Input: part model. Units: mm. Frame: model coordinates. Face numbers are marked on the shaded views. A direction names the side the tool comes from. Coordinates: 2 decimals unless noted, no trailing zeros. Order: outer loops, then holes, each group sorted by start corner. A loop starts at its lowest first (then second) coordinate and runs counter-clockwise, first axis right, second up.
from build123d import *

# Parameters (mm, degrees)
BASE_FLANGE1_DEPTH           = 3.175
EDGE_FLANGE1_DEPTH           = 16.378
EDGE_FLANGE2_STRIP_W         = 14.1732
EDGE_FLANGE2_STRIP_H         = 3.175
EDGE_FLANGE2_STRIP_CUT_DEPTH = 16.378
EDGE_FLANGE2_DEPTH           = 16.378
M5_CLEARANCE_HOLE1_D         = 5.5
M6_CLEARANCE_HOLE1_D         = 6.6
FILLET1_R                    = 2.54
M3_CLEARANCE_HOLE1_D         = 3.4


# Sheet-metal steps are written as plain solids
with BuildPart() as part:
    # Sketch1 → Base-Flange1 (new body)
    with BuildSketch(Plane.XY):
        Polygon((-22.215900005, -29.184600001), (-22.215900005, -69.692600001), (-5.837899995, -69.692600001), (-5.837899995, -45.562600001), (61.9125, -45.562600001), (61.9125, -29.184600001), align=None)
    extrude(amount=-BASE_FLANGE1_DEPTH)

    # Edge-Flange1 section (across the edge) → Edge-Flange1 (add)
    with BuildSketch(Plane(origin=(62.6491, -45.562600001, 0), x_dir=(-1, 0, 0), z_dir=(0, 1, 0))):
        with BuildLine():
            Line((-3.175, 0.7366), (-3.175, 32.0779))
            Line((-3.175, 32.0779), (0, 32.0779))
            Line((0, 32.0779), (0, 0.7366))
            ThreePointArc((0, 0.7366), (0.215745145, 0.215745145), (0.7366, 0))
            Line((0.7366, 0), (0.7366, -3.175))
            ThreePointArc((0.7366, -3.175), (-2.029318885, -2.029318885), (-3.175, 0.7366))
        make_face()
    extrude(amount=EDGE_FLANGE1_DEPTH)

    # Edge-Flange2 strip (across the edge) → Edge-Flange2 strip cut (cut)
    with BuildSketch(Plane(origin=(65.8241, -29.184600001, 32.0779), x_dir=(0, 0, -1), z_dir=(0, -1, 0))):
        with Locations((-6.35, -1.5875)):
            Rectangle(EDGE_FLANGE2_STRIP_W, EDGE_FLANGE2_STRIP_H)
    extrude(amount=EDGE_FLANGE2_STRIP_CUT_DEPTH, mode=Mode.SUBTRACT)

    # Edge-Flange2 section (across the edge) → Edge-Flange2 (add)
    with BuildSketch(Plane(origin=(65.8241, -29.184600001, 32.0779), x_dir=(0, 0, -1), z_dir=(0, -1, 0))):
        with BuildLine():
            Line((-3.175, 0.7366), (-3.175, 60.325))
            Line((-3.175, 60.325), (0, 60.325))
            Line((0, 60.325), (0, 0.7366))
            ThreePointArc((0, 0.7366), (0.215745145, 0.215745145), (0.7366, 0))
            Line((0.7366, 0), (0.7366, -3.175))
            ThreePointArc((0.7366, -3.175), (-2.029318885, -2.029318885), (-3.175, 0.7366))
        make_face()
    extrude(amount=EDGE_FLANGE2_DEPTH)

    # M5 Clearance Hole1 (through all)
    with Locations(Plane.XY.offset(35.2529)):
        with Locations((119.7991, -37.373600001)):
            Hole(M5_CLEARANCE_HOLE1_D / 2)

    # M6 Clearance Hole1 (through all)
    with Locations(Plane.XY):
        with Locations((-14.0269, -61.865600001)):
            Hole(M6_CLEARANCE_HOLE1_D / 2)

    # Fillet1
    fillet1_edges = [part.edges().sort_by_distance(p)[0] for p in [
        (-22.215900005, -69.692600001, -1.5875),
        (-22.215900005, -29.184600001, -1.5875),
        (-5.837899995, -45.562600001, -1.5875),
        (-5.837899995, -69.692600001, -1.5875),
        (126.1491, -29.184600001, 33.6654),
        (126.1491, -45.562600001, 33.6654),
    ]]
    fillet(fillet1_edges, radius=FILLET1_R)

    # M3 Clearance Hole1 (through all)
    with Locations(Plane.XY.offset(35.2529)):
        with Locations((96.0232, -37.423600001)):
            Hole(M3_CLEARANCE_HOLE1_D / 2)


solid = part.part
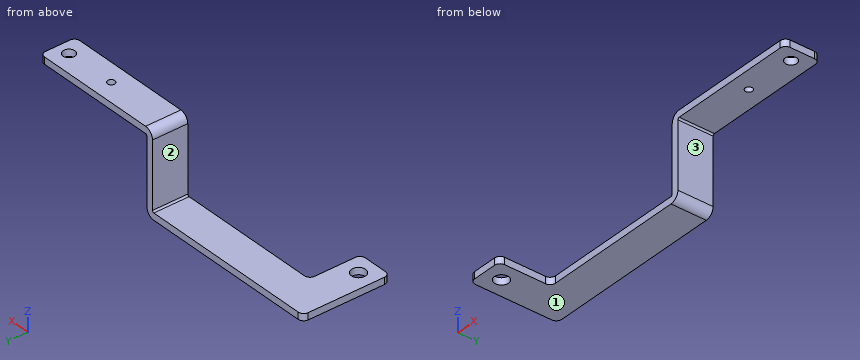
Item 1: Cut plane B-B on z = 25. Return loops of the section in (x, y).
Response values:
outline: (62.65, -45.56) - (65.82, -45.56) - (65.82, -29.18) - (62.65, -29.18) - close
Item 2: Pin query (flat end, axial travel): pin 1 Ø1 at (y, z) = (-56, -1) entering from +X; pin 2 Ø20.5 at (x, y) = (41, -55.5) entering from +Z; pin 3 Ø8 at (y, z) = (-33.5, 19.5) entering from -X. Return the tip coordinate at first contact, or that it passes through.
Response values:
pin 1: stops at x = -5.84
pin 2: stops at z = 0
pin 3: stops at x = 62.65
Item 3: Ray query, probe 1 along Z at (x, y) = (81.5, -41.5); probe 2 along Z at (x, y) = (34, -44) (3 decimals); probe 3 along X at (y, z) = (-42, 23.5). Return the intervals inside material, ascending.
Response values:
probe 1: z = 32.08 to 35.25
probe 2: z = -3.175 to 0
probe 3: x = 62.65 to 65.82
Item 4: Cut plane A-A on x = 96. Return loops of the section in (y, z), then the cut area to 3 significant figures.
Response values:
outline: (-45.56, 32.08) - (-39.12, 32.08) - (-39.12, 35.25) - (-45.56, 35.25) - close; (-35.72, 32.08) - (-29.18, 32.08) - (-29.18, 35.25) - (-35.72, 35.25) - close
area: 41.2 mm2
Item 5: Cut plane C-C on y = -56. Return loops of the section in (x, z) (3 decimals).
Response values:
outline: (-22.216, -3.175) - (-5.838, -3.175) - (-5.838, 0) - (-22.216, 0) - close
Item 6: Access query for the marked faces 1, 2 and 3. Directions: +Z, -Z, +X, -X, +Y, -Y. A direction counts if a zero-diameter tool reaches every point of the face in a straight line with its end or side. Return the directions, or none.
Response values:
face 1: -Z, +X, -X, +Y, -Y
face 2: +Z, -X, +Y, -Y
face 3: -Z, +X, +Y, -Y
